CAD build for the part. Positions are in the model's coordinates, mm. Give positions to 0.01 mm unless a question says otherwise; leave off trailing zeros. Loops run counter-clockwise (first coordinate to the right, second up) from the corner with the lowest first, then second, coordinate; pieces in that order, holes last. Notation, with made-up numbers: M 59,1.25 L 75,1.25 A6 cw 75,11.25 Z; hole C -11.75,67.25 d5. An arc over 180 degrees is marked long. One line per question, with ' | ' between items.
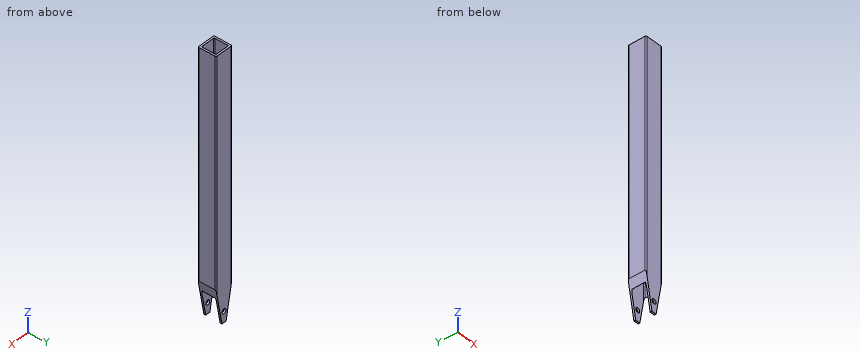
```python
from build123d import *

# Parameters (mm, degrees)
BOSS_EXTRUDE1_DEPTH      = 457.2
BOSS_EXTRUDE1_DEPTH_BACK = 457.2
SKETCH6_R                = 7.9375
CUT_EXTRUDE1_DEPTH       = 463.679319291


with BuildPart() as part:
    # Sketch4 → Boss-Extrude1 (new, two sides: drawn at the far end of the back side and taken through both)
    with BuildSketch(Plane.XY.offset(-BOSS_EXTRUDE1_DEPTH_BACK)):
        with BuildLine():
            Line((31.75, -28.575), (31.75, 28.575))
            ThreePointArc((31.75, 28.575), (30.82006403, 30.82006403), (28.575, 31.75))
            Line((28.575, 31.75), (-28.575, 31.75))
            ThreePointArc((-28.575, 31.75), (-30.82006403, 30.82006403), (-31.75, 28.575))
            Line((-31.75, 28.575), (-31.75, -28.575))
            ThreePointArc((-31.75, -28.575), (-30.82006403, -30.82006403), (-28.575, -31.75))
            Line((-28.575, -31.75), (28.575, -31.75))
            ThreePointArc((28.575, -31.75), (30.82006403, -30.82006403), (31.75, -28.575))
        make_face()
        with BuildLine():
            Line((25.4, 22.86), (25.4, -22.86))
            ThreePointArc((25.4, -22.86), (24.656051224, -24.656051224), (22.86, -25.4))
            Line((22.86, -25.4), (-22.86, -25.4))
            ThreePointArc((-22.86, -25.4), (-24.656051224, -24.656051224), (-25.4, -22.86))
            Line((-25.4, -22.86), (-25.4, 22.86))
            ThreePointArc((-25.4, 22.86), (-24.656051224, 24.656051224), (-22.86, 25.4))
            Line((-22.86, 25.4), (22.86, 25.4))
            ThreePointArc((22.86, 25.4), (24.656051224, 24.656051224), (25.4, 22.86))
        make_face(mode=Mode.SUBTRACT)
    extrude(amount=BOSS_EXTRUDE1_DEPTH + BOSS_EXTRUDE1_DEPTH_BACK)

    # Sketch6 → Cut-Extrude1 (cut, through all)
    with BuildSketch(Plane(origin=(0, 31.75, 0), x_dir=(1, 0, 0), z_dir=(0, 1, 0))):
        with Locations(Location((0, 419.1, 0), (0, 0, 270))):
            Circle(SKETCH6_R)
        Polygon((8.255, 457.2), (31.75, 330.2), (31.75, 457.2), align=None)
        Polygon((-8.255, 457.2), (-31.75, 330.2), (-31.75, 457.2), align=None)
    extrude(amount=-CUT_EXTRUDE1_DEPTH, mode=Mode.SUBTRACT)


solid = part.part
```
Item 1: Drill centre lines: line 1 along X through (y, z) = (-8, -264.5); line 2 along X through (y, z) = (28.5, -419.1). Where is each one in solid material? Low to high. Write a range as [from, to].
Conclusion:
line 1: [-31.75, -25.4], [25.4, 31.75] | line 2: [-15.3, -7.94], [7.94, 15.3]
Item 2: Saw through at D-D on z = -419.1. Give the cut face in (x, y), and give its area (3 significant figures).
Conclusion:
outline: M -15.3,-31.75 L -7.94,-31.75 L -7.94,-25.4 L -15.3,-25.4 Z; M -15.3,25.4 L -7.94,25.4 L -7.94,31.75 L -15.3,31.75 Z; M 7.94,-31.75 L 15.3,-31.75 L 15.3,-25.4 L 7.94,-25.4 Z; M 7.94,25.4 L 15.3,25.4 L 15.3,31.75 L 7.94,31.75 Z | area: 187 mm²
Item 3: Saw through at B-B on z = -320. Give the cut face in (x, y) (3 decimals), and give its area (3 significant figures).
Conclusion:
outline: M -31.75,-28.575 A3.175 ccw -28.575,-31.75 L 28.575,-31.75 A3.175 ccw 31.75,-28.575 L 31.75,28.575 A3.175 ccw 28.575,31.75 L -28.575,31.75 A3.175 ccw -31.75,28.575 Z; hole M -25.4,-22.86 A2.54 ccw -22.86,-25.4 L 22.86,-25.4 A2.54 ccw 25.4,-22.86 L 25.4,22.86 A2.54 ccw 22.86,25.4 L -22.86,25.4 A2.54 ccw -25.4,22.86 Z | area: 1,450 mm²
Item 4: Saw through at A-A on y = 5.5. Give the cut face in (x, z).
Conclusion:
outline: M -31.75,-330.2 L -25.4,-364.52 L -25.4,457.2 L -31.75,457.2 Z; M 25.4,-364.52 L 31.75,-330.2 L 31.75,457.2 L 25.4,457.2 Z
Item 5: Saw through at C-C on x = 0. Give the cut face in (y, z).
Conclusion:
outline: M -31.75,-457.2 L -25.4,-457.2 L -25.4,-427.04 L -31.75,-427.04 Z; M -31.75,-411.16 L -25.4,-411.16 L -25.4,457.2 L -31.75,457.2 Z; M 25.4,-457.2 L 31.75,-457.2 L 31.75,-427.04 L 25.4,-427.04 Z; M 25.4,-411.16 L 31.75,-411.16 L 31.75,457.2 L 25.4,457.2 Z
Item 6: Drop flat-ended pins along their axis: P1, Ø14.5, axis at x = 0, z = -419.1, coming from the -Y side; P2, Ø20.5, axis at x = 0, z = -419.1, coming from the -Y side. Give the stop position or say it passes through.
Conclusion:
P1: through | P2: y = -31.75
